Verification items for this drawing (mm, ordinates from the low corner). Round coordinates to 2 decimals unless told otherwise and drop trailing zeros. Write each loop counter-clockwise with the first axis right and the second up, starting at its lowest first coordinate (ties: lowest second). Pieces come first, ordered by that corner, then holes. Notation, with made-up numbers: M 7,74.5 L 40,74.5 A12 ccw 40,96.5 Z; hole C 57.25,31 d8. An arc over 180 degrees is marked long. Write each question's results on one line, items separated by ' | '.
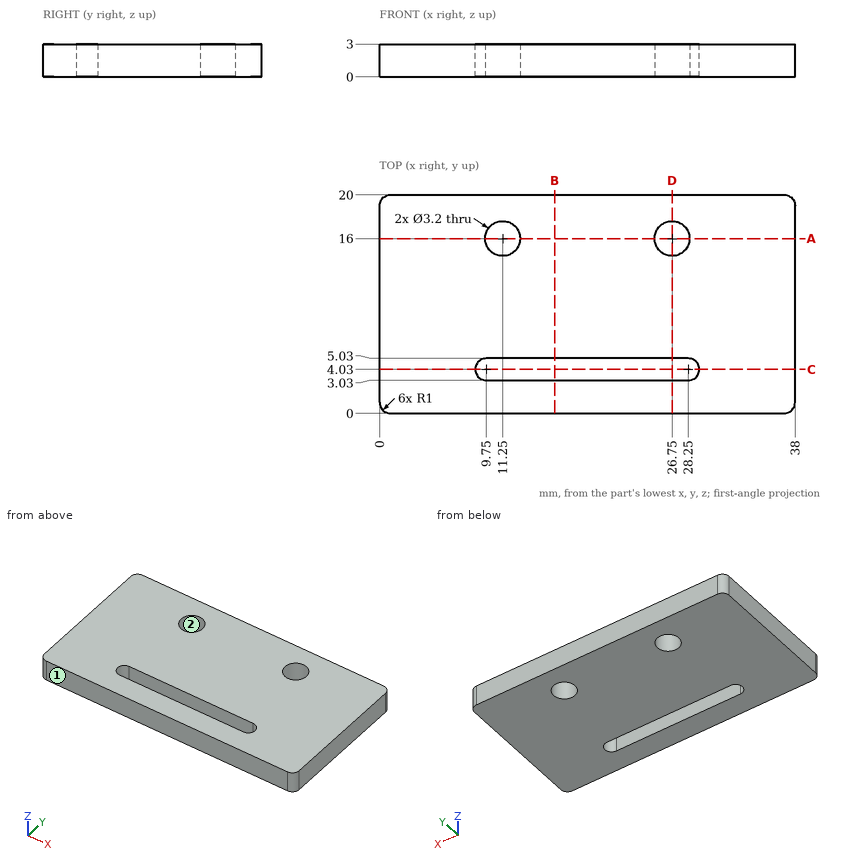
1) Sectioned sample at C-C, the plane y = 4.03. Record the cut outline in (x, z), and give its area (3 significant figures).
Calculated:
outline: M 0,0 L 8.75,0 L 8.75,3 L 0,3 Z; M 29.25,0 L 38,0 L 38,3 L 29.25,3 Z | area: 52.5 mm²
2) Draft check along X on the marked faces 1 and 2. Enter one of: pulls with the +X half, pulls with the -X half, needs draft (parallel to the pull), parting line crosses it, or undercut.
Calculated:
face 1: needs draft | face 2: undercut
3) Sectioned sample at B-B, the plane x = 16. Record the cut outline in (y, z).
Calculated:
outline: M 0,0 L 3.03,0 L 3.03,3 L 0,3 Z; M 5.03,0 L 20,0 L 20,3 L 5.03,3 Z
4) Sectioned sample at A-A, the plane y = 16. Record the cut outline in (x, z), and give its area (3 significant figures).
Calculated:
outline: M 0,0 L 9.65,0 L 9.65,3 L 0,3 Z; M 12.85,0 L 25.15,0 L 25.15,3 L 12.85,3 Z; M 28.35,0 L 38,0 L 38,3 L 28.35,3 Z | area: 94.8 mm²
5) Sectioned sample at D-D, the plane x = 26.75. Record the cut outline in (y, z), and give its area (3 significant figures).
Calculated:
outline: M 0,0 L 3.03,0 L 3.03,3 L 0,3 Z; M 5.03,0 L 14.4,0 L 14.4,3 L 5.03,3 Z; M 17.6,0 L 20,0 L 20,3 L 17.6,3 Z | area: 44.4 mm²
6) Material ranges on line 1 (Y direction, x = 26.75, z = 1.3); line 2 (X direction, y = 16.5, z = 2.25); line 3 (Y direction, x = 20.5, z = 1.4), recorded low to high. Write a range as [from, to].
Calculated:
line 1: y = [0, 3.03], [5.03, 14.4], [17.6, 20] | line 2: x = [0, 9.73], [12.77, 25.23], [28.27, 38] | line 3: y = [0, 3.03], [5.03, 20]
